from build123d import *

# Parameters (mm, degrees)
ESBO_O7_R                  = 22
RESSALTO_EXTRUS_O1_DEPTH   = 46
ESBO_O11_R                 = 17.8
CORTE_EXTRUS_O1_DEPTH      = 43
CORTE_EXTRUS_O3_DEPTH      = 56.533773508
CORTE_EXTRUS_O3_DEPTH_BACK = 56.533773508
ESBO_O15_R                 = 4.75


with BuildPart() as part:
    # Esboço7 → Ressalto-extrusão1 (new body)
    with BuildSketch(Plane.XY):
        Circle(ESBO_O7_R)
    extrude(amount=RESSALTO_EXTRUS_O1_DEPTH)

    # Esboço11 → Corte-extrusão1 (cut)
    with BuildSketch(Plane.XY):
        Circle(ESBO_O11_R)
    extrude(amount=CORTE_EXTRUS_O1_DEPTH, mode=Mode.SUBTRACT)

    # Esboço15 → Corte-extrusão3 (cut, two sides: drawn at the far end of the back side and taken through both)
    with BuildSketch(Plane(origin=(0, 0, 0), x_dir=(1, 0, 0), z_dir=(0, 1, 0)).offset(-CORTE_EXTRUS_O3_DEPTH_BACK)):
        with Locations(Location((0, -24.505035598, 0), (0, 0, 270))):
            Circle(ESBO_O15_R)
    extrude(amount=CORTE_EXTRUS_O3_DEPTH + CORTE_EXTRUS_O3_DEPTH_BACK, mode=Mode.SUBTRACT)


solid = part.part
Source: CAD feature listing. Evaluate the final solid. Frame: model axes, mm. A direction names the side the tool comes from. Round coordinates to 2 decimals unless told otherwise and drop trailing zeros. Write each loop counter-clockwise with the first axis right and the second up, starting at its lowest first coordinate (ties: lowest second). Pieces come first, ordered by that corner, then holes. Notation, with made-up numbers: (-32.5, 49.25) - (-17.5, 49.25) arc R16 ccw to (-17.5, 65.25) - close; hole circle Ø1 at (87, -17.75). An arc over 180 degrees is marked (long way). Use CSV: the item, a comma, the result in double quotes. Start each with the question number.
(1) First-contact query: pin 1 Ø6 at (y, z) = (-4, 21) entering from -X; pin 2 Ø4 at (x, z) = (-13, 31.5) entering from -Y; pin 3 Ø1 at (x, z) = (2, 17) entering from +Y. Flat tips, straight axial feed; report the tip coordinate or a pass-through.
(2) Cut plane A-A, the plane x = 0. Return loops of the section in (y, z).
(3) Cut plane C-C, the plane y = -9.5. Return loops of the section in (x, z), and give its area (3 significant figures).
(4) Mould query, pull axis X, two halves, no side actions, for faces 3 (the face through (0, 0, 46)), 4 (the face through (-4.769, -21.477, 22.678)), 5 (the face through (-1.8, -19.6, 28.9)). Classes: pulls with the +X half, pulls with the -X half, needs draft (parallel to the pull), parting line crosses it, or undercut.
(5) Cut plane D-D, the plane x = -6. Return loops of the section in (y, z).
(6) Cut plane B-B, the plane z = 12.5. Return loops of the section in (x, y).
(7) Material intervals for probe 1 along Y at (x, z) = (0, 11); probe 2 along Z at (x, y) = (0, 20.1); probe 3 along Z at (x, y) = (-10.5, 3.5), sorted ascending. Write a range as [from, to].
(8) Set-up query: faces 1 (the face through (0, 0, 43)), 2 (the face through (18, 0, 0)). Return all of +Z, -Z, +X, -X, +Y, -Y with unobstructed straight access to the full face (end or side cutting, diameter ignored); none if empty.
Geometry says:
1,pin 1,"x = -21.98"
1,pin 2,"y = -19.05"
1,pin 3,"y = 21.95"
2,outline,"(-22, 0) - (-17.8, 0) - (-17.8, 19.76) - (-22, 19.76) - close; (-22, 29.26) - (-17.8, 29.26) - (-17.8, 43) - (17.8, 43) - (17.8, 29.26) - (22, 29.26) - (22, 46) - (-22, 46) - close; (17.8, 0) - (22, 0) - (22, 19.76) - (17.8, 19.76) - close"
3,outline,"(-19.84, 0) - (-15.05, 0) - (-15.05, 43) - (15.05, 43) - (15.05, 0) - (19.84, 0) - (19.84, 46) - (-19.84, 46) - close"
3,area,"531 mm²"
4,face 3,"needs draft"
4,face 4,"parting line crosses it"
4,face 5,"undercut"
5,outline,"(-21.17, 0) - (-16.76, 0) - (-16.76, 43) - (16.76, 43) - (16.76, 0) - (21.17, 0) - (21.17, 46) - (-21.17, 46) - close"
6,outline,"circle Ø44 at (0, 0); hole circle Ø35.6 at (0, 0)"
7,probe 1,"[-22, -17.8], [17.8, 22]"
7,probe 2,"[0, 19.76], [29.26, 46]"
7,probe 3,"[43, 46]"
8,face 1,"-Z"
8,face 2,"-Z, +X, -X, +Y, -Y"
